Input: part model. Units: mm. Frame: model coordinates. Face numbers are marked on the shaded views. A direction names the side the tool comes from. Give positions to 0.01 mm unless a question says otherwise; leave off trailing zeros. Loops run counter-clockwise (first coordinate to the right, second up) from the corner with the lowest first, then second, coordinate; pieces in that order, holes last. Notation, with made-up numbers: (-7, -35.5) -> (24, -35.5) arc R14 cw to (24, -11.5) -> close; hole circle Ø8 at (82.25, -5.75). An arc over 180 degrees is marked (long way). Answer as a JSON object with one key per item and string values. Group by question number.
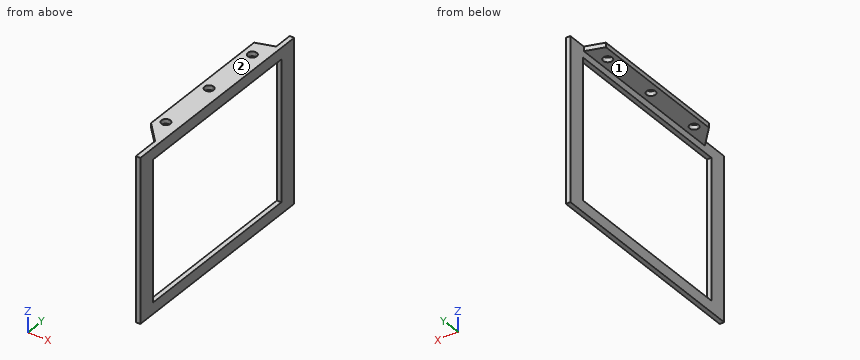
```python
from build123d import *

# Parameters (mm, degrees)
F0_W     = 3.175
F0_H     = 152.4
F1_DEPTH = 114.3
F2_W     = 127
F2_H     = 98.425
F3_DEPTH = 25.4
F4_W     = 119.8984608054
F4_H     = 3.175
F5_DEPTH = 12.7
F7_DEPTH = 25.4
F9_DEPTH = 25.4


with BuildPart() as f1:
    # F0 (on Top) → F1 (new body)
    with BuildSketch(Plane.XY):
        Rectangle(F0_W, F0_H)
    extrude(amount=F1_DEPTH)

    # F2 (on face) → F3 (cut)
    with BuildSketch(Plane.YZ.offset(1.5875)):
        with Locations((0, 57.15)):
            Rectangle(F2_W, F2_H)
    extrude(amount=-F3_DEPTH, mode=Mode.SUBTRACT)

    # F4 (on face) → F5 (join)
    with BuildSketch(Plane(origin=(-1.5875, 0, 0), x_dir=(0, -1, 0), z_dir=(-1, 0, 0))):
        with Locations((-2.8692372143, 112.7125)):
            Rectangle(F4_W, F4_H)
    extrude(amount=F5_DEPTH)

    # F6 (on face) → F7 (cut)
    with BuildSketch(Plane.XY.offset(114.3)):
        Polygon((-14.2875, 58.8119849563), (-1.5875, 62.818467617), (-14.2875, 62.818467617), align=None)
        Polygon((-14.2875, -57.0799931884), (-1.5875, -57.0799931884), (-14.2875, -43.1980900466), align=None)
    extrude(amount=-F7_DEPTH, mode=Mode.SUBTRACT)

    # F8 (on face) → F9 (cut)
    with BuildSketch(Plane.XY.offset(114.3)):
        with BuildLine():
            ThreePointArc((-4.7625, 48.1152262866), (-5.6924359697, 50.3602903169), (-7.9375, 51.2902262866))
            Line((-7.9375, 51.2902262866), (-7.9375, 44.9402262866))
            ThreePointArc((-7.9375, 44.9402262866), (-5.6924359697, 45.8701622564), (-4.7625, 48.1152262866))
        make_face()
        with BuildLine():
            ThreePointArc((-4.7625, -37.4390416175), (-5.6924359697, -35.1939775872), (-7.9375, -34.2640416175))
            Line((-7.9375, -34.2640416175), (-7.9375, -40.6140416175))
            ThreePointArc((-7.9375, -40.6140416175), (-5.6924359697, -39.6841056478), (-4.7625, -37.4390416175))
        make_face()
        with BuildLine():
            Line((-7.9375, -40.6140416175), (-7.9375, -34.2640416175))
            ThreePointArc((-7.9375, -34.2640416175), (-11.1125, -37.4390416175), (-7.9375, -40.6140416175))
        make_face()
        with BuildLine():
            ThreePointArc((-4.7625, 5.3380923346), (-5.6924359697, 7.5831563648), (-7.9375, 8.5130923346))
            Line((-7.9375, 8.5130923346), (-7.9375, 2.1630923346))
            ThreePointArc((-7.9375, 2.1630923346), (-5.6924359697, 3.0930283043), (-4.7625, 5.3380923346))
        make_face()
        with BuildLine():
            Line((-7.9375, 2.1630923346), (-7.9375, 8.5130923346))
            ThreePointArc((-7.9375, 8.5130923346), (-11.1125, 5.3380923346), (-7.9375, 2.1630923346))
        make_face()
        with BuildLine():
            Line((-7.9375, 44.9402262866), (-7.9375, 51.2902262866))
            ThreePointArc((-7.9375, 51.2902262866), (-11.1125, 48.1152262866), (-7.9375, 44.9402262866))
        make_face()
    extrude(amount=-F9_DEPTH, mode=Mode.SUBTRACT)


solid = f1.part
```
Q1. Ray query, probe 1 along Z at (x, y) = (0.25, 2); probe 2 along Y at (x, z) = (-0.5, 55); probe 3 along Z at (x, y) = (-2.25, -34.5) (3 decimals). Return the intervals inside material, ascending.
Q2. Section B-B on z = 26.5. Return the cut outline in (x, y), then the cut area to 3 significant figures.
Q3. Section C-C on y = -45.5. Return the cut outline in (x, z) (1 decimal), then the cut area to 3 significant figures.
Q4. Section D-D on y = 67.5. Return the cut outline in (x, z).
Q5. Section A-A on y = -23.5. Return the cut outline in (x, z) (1 decimal), then the cut area to 3 significant figures.
Q6. Set-up query: the marked faces 1 and 2. Return all of +Z, -Z, +X, -X, +Y, -Y with unobstructed straight access to the full face (end or side cutting, diameter ignored); none if empty.
Numbers:
{
 "1": {"probe 1": "z = 0 to 7.94, 106.36 to 114.3", "probe 2": "y = -76.2 to -63.5, 63.5 to 76.2", "probe 3": "z = 111.125 to 114.3"},
 "2": {"outline": "(-1.59, -76.2) -> (1.59, -76.2) -> (1.59, -63.5) -> (-1.59, -63.5) -> close; (-1.59, 63.5) -> (1.59, 63.5) -> (1.59, 76.2) -> (-1.59, 76.2) -> close", "area": "80.6 mm²"},
 "3": {"outline": "(-12.2, 111.1) -> (-1.6, 111.1) -> (-1.6, 106.4) -> (1.6, 106.4) -> (1.6, 114.3) -> (-12.2, 114.3) -> close; (-1.6, 0) -> (1.6, 0) -> (1.6, 7.9) -> (-1.6, 7.9) -> close", "area": "84.0 mm²"},
 "4": {"outline": "(-1.59, 0) -> (1.59, 0) -> (1.59, 114.3) -> (-1.59, 114.3) -> close"},
 "5": {"outline": "(-14.3, 111.1) -> (-1.6, 111.1) -> (-1.6, 106.4) -> (1.6, 106.4) -> (1.6, 114.3) -> (-14.3, 114.3) -> close; (-1.6, 0) -> (1.6, 0) -> (1.6, 7.9) -> (-1.6, 7.9) -> close", "area": "90.7 mm²"},
 "6": {"face 1": "-Z, -X, +Y, -Y", "face 2": "+Z, +X, -X, +Y, -Y"}
}
